Input: part model. Units: mm. Frame: model coordinates. Face numbers are marked on the shaded views. A direction names the side the tool comes from. Round coordinates to 2 decimals unless told otherwise and drop trailing zeros. Loops run counter-clockwise (first coordinate to the right, second up) from the corner with the lowest first, then second, coordinate; pieces in that order, holes last. Notation, with made-up numbers: (-11, 52.25) -> (29, 52.25) arc R12 ccw to (29, 75.25) -> close; hole circle Ø11 at (20.25, -38). An arc over 180 degrees is marked (long way). Answer as a JSON object with one key per item and string values.
Autodesk Inventor part; units mm, degrees
ref_plane "YZ Plane" through (0, 0, 0) normal (1, 0, 0) x (0, 1, 0)
ref_plane "XZ Plane" through (0, 0, 0) normal (0, 1, 0) x (-1, 0, 0)
ref_plane "XY Plane" through (0, 0, 0) normal (0, 0, 1) x (1, 0, 0)
sketch "Sketch1" plane through (0, 0, 0) normal (0, 0, 1) x (1, 0, 0)
  circle A0 centre (0, 0) radius 25.4
  circle A1 centre (0, 19.05) radius 2.0828
  line L0 (0, 0) -> (0, 19.05) construction
  circle A2 centre (-16.4978, 9.525) radius 2.0828
  circle A3 centre (-16.4978, -9.525) radius 2.0828
  circle A4 centre (0, -19.05) radius 2.0828
  circle A5 centre (16.4978, -9.525) radius 2.0828
  circle A6 centre (16.4978, 9.525) radius 2.0828
  line L1 (6.858, -3.9595) -> (0, -7.9189)
  line L2 (0, -7.9189) -> (-6.858, -3.9595)
  line L3 (-6.858, -3.9595) -> (-6.858, 3.9595)
  line L4 (-6.858, 3.9595) -> (0, 7.9189)
  line L5 (0, 7.9189) -> (6.858, 3.9595)
  line L6 (6.858, 3.9595) -> (6.858, -3.9595)
  dimension "d0" = 50.8
  dimension "d2" = 4.1656
  dimension "d3" = 19.05
  dimension "d6" = 360
  dimension "d10" = 13.716
extrude "Extrusion1" add sketch "Sketch1" along normal blind 3.175
properties part number "Hex Shaft Connector (Lexan)" material "Aluminum 6061"
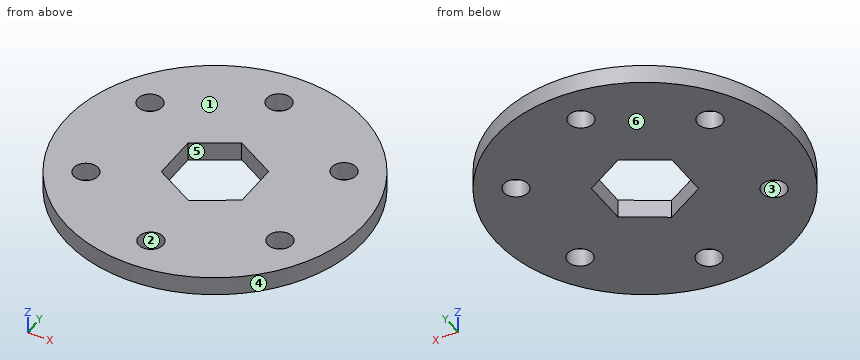
1) Section D-D, the plane z = 1.45. Count the separate pieces of the cut face and the enclosed holes in it, plus the area to 3 significant figures.
Output:
{"separate pieces": "1", "enclosed holes": "7", "area": "1,780 mm^2"}
2) Section C-C, the plane y = 11. Output: boundary loops of the cut face in (x, z) (3 decimals), plus the area to 3 significant figures.
Output:
{"outline": "(-22.895, 0) -> (-17.968, 0) -> (-17.968, 3.175) -> (-22.895, 3.175) -> close; (-15.027, 0) -> (15.027, 0) -> (15.027, 3.175) -> (-15.027, 3.175) -> close; (17.968, 0) -> (22.895, 0) -> (22.895, 3.175) -> (17.968, 3.175) -> close", "area": "127 mm^2"}
3) Section A-A, the plane y = 19.05. Output: boundary loops of the cut face in (x, z) (3 decimals), plus the area to 3 significant figures.
Output:
{"outline": "(-16.801, 0) -> (-2.083, 0) -> (-2.083, 3.175) -> (-16.801, 3.175) -> close; (2.083, 0) -> (16.801, 0) -> (16.801, 3.175) -> (2.083, 3.175) -> close", "area": "93.5 mm^2"}
4) Reachability of the marked faces 5 and 6 from +Z, -Z, +X, -X, +Y, -Y: full face, straight path, thin tool, end or side. Return the list, or none.
Output:
{"face 5": "+Z, -Z", "face 6": "-Z, +X, -X, +Y, -Y"}
5) Section B-B, the plane x = -3.5. Output: boundary loops of the cut face in (y, z) (3 decimals).
Output:
{"outline": "(-25.158, 0) -> (-5.898, 0) -> (-5.898, 3.175) -> (-25.158, 3.175) -> close; (5.898, 0) -> (25.158, 0) -> (25.158, 3.175) -> (5.898, 3.175) -> close"}
6) Draft query along X for the marked faces 1, 2, 3 and 4. Return one class per face: +X half, -X half, draft (parallel to the pull), parting line (faces both ways), or undercut.
Output:
{"face 1": "draft", "face 2": "undercut", "face 3": "undercut", "face 4": "parting line"}
7) Ray query, probe 1 along Y at (x, z) = (0, 2.3); probe 2 along X at (y, z) = (9, 2.4); probe 3 along X at (y, z) = (-18.5, 2.7). Return the intervals inside material, ascending.
Output:
{"probe 1": "y = -25.4 to -21.13, -16.97 to -7.92, 7.92 to 16.97, 21.13 to 25.4", "probe 2": "x = -23.75 to -18.51, -14.48 to 14.48, 18.51 to 23.75", "probe 3": "x = -17.4 to -2.01, 2.01 to 17.4"}
